Geometry check sheet. Reference: the model listing, model coordinates, mm. A direction names the side the tool comes from. Round coordinates to 2 decimals unless told otherwise and drop trailing zeros. Order: outer loops, then holes, each group sorted by start corner. A loop starts at its lowest first (then second) coordinate and runs counter-clockwise, first axis right, second up. Notation, with made-up numbers: (36.5, -0.5) - (95.5, -0.5) arc R25 ccw to (95.5, 38.5) - close; hole circle Ø5 at (34, -25.5). An arc over 180 degrees is marked (long way). Answer as CSV lines item,"result". Start each with the question number.
```python
from build123d import *

# Parameters (mm, degrees)
ESQUISSE1_W                    = 120
ESQUISSE1_H                    = 215
BOSS_EXTRU_1_DEPTH             = 6
ESQUISSE2_R                    = 1.6
ENL_V_MAT_EXTRU_1_DEPTH        = 138.798088748
R_P_TITION_LIN_AIRE1_OUTLINE_R = 1.6
R_P_TITION_LIN_AIRE1_DEPTH     = 6
ESQUISSE3_W                    = 38
ESQUISSE3_H                    = 23
ESQUISSE3_W_2                  = 18.381114661
ESQUISSE3_H_2                  = 18.590181779
ENL_V_MAT_EXTRU_2_DEPTH        = 138.798088748
ENL_V_MAT_EXTRU_3_DEPTH        = 138.798088748
CONG_1_R                       = 5
ESQUISSE5_R                    = 1.6
ENL_V_MAT_EXTRU_4_DEPTH        = 10
ESQUISSE6_W                    = 56
ESQUISSE6_H                    = 30
ENL_V_MAT_EXTRU_5_DEPTH        = 138.798088748


# Read off the part's stored shape, not the designer's step: Répétition linéaire1
with BuildPart() as part:
    # Esquisse1 → Boss.-Extru.1 (new body)
    with BuildSketch(Plane.XY):
        with Locations((22.778700537, 2.5)):
            Rectangle(ESQUISSE1_W, ESQUISSE1_H)
    extrude(amount=BOSS_EXTRU_1_DEPTH)

    # Esquisse2 → Enlèv. mat.-Extru.1 (cut, through all)
    with BuildSketch(Plane.XY.offset(6)):
        with Locations((-27.221299463, -60)):
            Circle(ESQUISSE2_R)
    extrude(amount=-ENL_V_MAT_EXTRU_1_DEPTH, mode=Mode.SUBTRACT)

    # Répétition linéaire1 outline → Répétition linéaire1 (cut)
    with BuildSketch(Plane.XY):
        with Locations((-27.221299463, -10)):
            Circle(R_P_TITION_LIN_AIRE1_OUTLINE_R)
        with Locations((-22.221299463, 40)):
            Circle(R_P_TITION_LIN_AIRE1_OUTLINE_R)
        with Locations((-17.221299463, 90)):
            Circle(R_P_TITION_LIN_AIRE1_OUTLINE_R)
        with Locations((22.778700537, -60)):
            Circle(R_P_TITION_LIN_AIRE1_OUTLINE_R)
        with Locations((22.778700537, 15)):
            Circle(R_P_TITION_LIN_AIRE1_OUTLINE_R)
        with Locations((62.778700537, 90)):
            Circle(R_P_TITION_LIN_AIRE1_OUTLINE_R)
        with Locations((67.778700537, 40)):
            Circle(R_P_TITION_LIN_AIRE1_OUTLINE_R)
        with Locations((72.778700537, -10)):
            Circle(R_P_TITION_LIN_AIRE1_OUTLINE_R)
        with Locations((72.778700537, -60)):
            Circle(R_P_TITION_LIN_AIRE1_OUTLINE_R)
        with Locations((22.778700537, 90)):
            Circle(R_P_TITION_LIN_AIRE1_OUTLINE_R)
    extrude(amount=R_P_TITION_LIN_AIRE1_DEPTH, mode=Mode.SUBTRACT)

    # Esquisse3 → Enlèv. mat.-Extru.2 (cut, through all)
    with BuildSketch(Plane(origin=(0, 0, 0), x_dir=(-1, 0, 0), z_dir=(0, 0, -1))):
        with Locations((0.408750369, -17.5)):
            Rectangle(ESQUISSE3_W, ESQUISSE3_H)
        with Locations((-7.196798698, -54.48972052)):
            Rectangle(ESQUISSE3_W_2, ESQUISSE3_H_2)
        with BuildLine():
            Line((4.557875847, 36.021320392), (-13.074694363, 36.021320392))
            ThreePointArc((-13.074694363, 36.021320392), (-20.807462052, 43.75408808), (-13.074694363, 51.486855768))
            Line((-13.074694363, 51.486855768), (4.557875847, 51.486855768))
            ThreePointArc((4.557875847, 51.486855768), (12.290643535, 43.75408808), (4.557875847, 36.021320392))
        make_face()
        Polygon((-51.286994849, -11.69900166), (-51.286994849, 40.852954993), (-70.100011596, 34.728797636), (-70.479177032, -6.090187837), align=None)
        with BuildLine():
            Line((-30.778700537, -101), (-30.778700537, -105))
            Line((-30.778700537, -105), (-14.778700537, -105))
            Line((-14.778700537, -105), (-14.778700537, -101))
            ThreePointArc((-14.778700537, -101), (-22.778700537, -93), (-30.778700537, -101))
        make_face()
    extrude(amount=-ENL_V_MAT_EXTRU_2_DEPTH, mode=Mode.SUBTRACT)

    # Esquisse4 → Enlèv. mat.-Extru.3 (cut, through all)
    with BuildSketch(Plane.XY.offset(6)):
        Polygon((-37.221299463, 110), (-37.221299463, 4.99999922), (-26.615238451, 110), align=None)
        Polygon((72.172639526, 110), (82.778700537, 110), (82.778700537, 4.99999922), align=None)
    extrude(amount=-ENL_V_MAT_EXTRU_3_DEPTH, mode=Mode.SUBTRACT)

    # Congé1
    cong_1_edges = [part.edges().sort_by_distance(p)[0] for p in [
        (70.100011596, 34.728797636, 3),
        (51.286994849, 40.852954993, 3),
        (51.286994849, -11.69900166, 3),
        (70.479177032, -6.090187837, 3),
    ]]
    fillet(cong_1_edges, radius=CONG_1_R)

    # Esquisse5 → Enlèv. mat.-Extru.4 (cut)
    with BuildSketch(Plane.XY.offset(6)):
        with Locations((67.778700537, -94.54)):
            Circle(ESQUISSE5_R)
    extrude(amount=-ENL_V_MAT_EXTRU_4_DEPTH, mode=Mode.SUBTRACT)

    # Esquisse6 → Enlèv. mat.-Extru.5 (cut, through all)
    with BuildSketch(Plane.XY.offset(6)):
        with Locations((22.778700537, -90)):
            Rectangle(ESQUISSE6_W, ESQUISSE6_H)
    extrude(amount=-ENL_V_MAT_EXTRU_5_DEPTH, mode=Mode.SUBTRACT)


solid = part.part
```
1. Access from +Z, -Z, +X, -X, +Y, -Y to the whole of each face (thin tool, end or side, straight path). Record for faces 1 (the face through (7, -45.195, 3)), 2 (the face through (82.779, -51, 3)), 3 (the face through (-5.221, -90, 3)).
2. Go/stop test with flat-tipped pins: pin 1 Ø2.5 at (x, y) = (72.78, -10) entering from +Z; pin 2 Ø3 at (x, z) = (5.5, 4) entering from -Y; pin 3 Ø1 at (y, z) = (34, 3.5) entering from -X. Record where each tip stops, or that it passes through.
3. Section check B-B on y = 79. Record the boundary of the cut face in (x, z).
4. Draft check along Y on faces 4 (the face through (62.33, -8.47, 2.96)), 5 (the face through (-21, -105, 3)), 6 (the face through (4, 36.021, 3)), 7 (the face through (77.55, 56.76, 3.04)). Enter one of: released by +Y, released by -Y, zero draft, split by the parting line, or undercut.
5. Thickness scan on probe 1 along X at (y, z) = (-94.54, 1.8); probe 2 along Y at (x, z) = (-2.5, 4.5); probe 3 along Y at (x, z) = (6, 0.7). Record the ranges inside material, lowest first.
6. Section check A-A on z = 2.95. Count the separate pieces of the cut face and the enclosed holes in it, plus the area to 3 significant figures.
Numbers:
1,face 1,"+Z, -Z"
1,face 2,"+Z, -Z, +X, +Y, -Y"
1,face 3,"+Z, -Z, -Y"
2,pin 1,"passes through"
2,pin 2,"stops at y = -75"
2,pin 3,"stops at x = -34.34"
3,outline,"(-29.75, 0) - (75.3, 0) - (75.3, 6) - (-29.75, 6) - close"
4,face 4,"undercut"
4,face 5,"released by -Y"
4,face 6,"undercut"
4,face 7,"released by +Y"
5,probe 1,"x = -37.22 to -5.22, 50.78 to 66.18, 69.38 to 82.78"
5,probe 2,"y = -75 to -29, -6 to 36.02, 51.49 to 110"
5,probe 3,"y = -75 to -63.78, -45.19 to -29, -6 to 36.02, 51.49 to 110"
6,separate pieces,"1"
6,enclosed holes,"16"
6,area,"20,400 mm2"
